Could you check a few things on this model? Use its own coordinates, in mm. A direction names the side the tool comes from. Give positions to 0.01 mm unless a question says otherwise; leave off trailing zeros. Write each loop counter-clockwise with the first axis right and the second up, starting at its lowest first coordinate (ties: lowest second). Pieces come first, ordered by that corner, then holes. Notation, with made-up numbers: (-36, 67.5) - (-30, 67.5) arc R29 ccw to (-30, 90.5) - close; hole circle Ø4 at (66.25, 58). An arc over 180 degrees is marked (long way). Answer as a JSON object with one key per item and string values. Group by question number.
```python
from build123d import *

# Parameters (mm, degrees)
SKETCH1_3_R                       = 260
SKETCH1_3_R_2                     = 240
BOSS_EXTRUDE1_DEPTH               = 180
BOSS_EXTRUDE2_DEPTH               = 20
BOSS_EXTRUDE3_DEPTH               = 20
CUT_EXTRUDE1_DEPTH                = 20
F_1_2_13_TAPPED_HOLE1_AT_2_COUNT  = 2
F_1_2_13_TAPPED_HOLE1_AT_2_PITCH  = 353.553390593
F_1_2_13_TAPPED_HOLE1_AT_3_COUNT  = 2
F_1_2_13_TAPPED_HOLE1_AT_3_PITCH  = 463.112622797
F_1_2_13_TAPPED_HOLE7_D           = 10.71626
F_1_2_13_TAPPED_HOLE7_DEPTH       = 45.9
F_1_2_13_TAPPED_HOLE7_CBORE_D     = 12.7
F_1_2_13_TAPPED_HOLE7_CBORE_DEPTH = 40
F_1_2_13_TAPPED_HOLE7_TIP         = 3.219489309


with BuildPart() as part:
    # Sketch1<3> → Boss-Extrude1 (new body)
    with BuildSketch(Plane(origin=(0, 0, 0), x_dir=(0, 0, -1), z_dir=(1, 0, 0))):
        with Locations(Location((0, 0, 0), (0, 0, 180))):
            Circle(SKETCH1_3_R)
        with Locations(Location((0, 0, 0), (0, 0, 180))):
            Circle(SKETCH1_3_R_2, mode=Mode.SUBTRACT)
    extrude(amount=BOSS_EXTRUDE1_DEPTH)

    # Sketch6 → Boss-Extrude2 (add)
    with BuildSketch(Plane(origin=(0, 0, 0), x_dir=(0, 0, -1), z_dir=(1, 0, 0))):
        with BuildLine():
            Line((-260, -40), (-260, -400))
            Line((-260, -400), (260, -400))
            Line((260, -400), (260, -40))
            Line((260, -40), (256.904651573, -40))
            ThreePointArc((256.904651573, -40), (0, -260), (-256.904651573, -40))
            Line((-256.904651573, -40), (-260, -40))
        make_face()
    extrude(amount=BOSS_EXTRUDE2_DEPTH)

    # Sketch11 → Boss-Extrude3 (add)
    with BuildSketch(Plane(origin=(150, 0, 0), x_dir=(0, 0, -1), z_dir=(1, 0, 0))):
        with BuildLine():
            Line((-260, -40), (-260, -400))
            Line((-260, -400), (260, -400))
            Line((260, -400), (260, -40))
            Line((260, -40), (256.904651573, -40))
            ThreePointArc((256.904651573, -40), (0, -260), (-256.904651573, -40))
            Line((-256.904651573, -40), (-260, -40))
        make_face()
    extrude(amount=-BOSS_EXTRUDE3_DEPTH)

    # Sketch23 → 1/2-13 Tapped Hole6 (revolve, cut)
    with BuildSketch(Plane(origin=(70.297889329, -259.97605488, 3.528581758), x_dir=(0, -0.013571468301340803, -0.9999079033831796), z_dir=(1, 0, 0))):
        Polygon((0, 0), (0, 33.219489309), (5.35813, 30), (5.35813, 40), (6.35, 40), (6.35, 0), align=None)
    revolve(axis=Axis((70.297889329, -266.325470066, 3.614760582), (0, 0.9999079033831795, -0.013571468301340804)), mode=Mode.SUBTRACT)

    # Sketch23 at point 2 (carried to point 2, square into its face) → 1/2-13 Tapped Hole6 at 2 (revolve, cut)
    with BuildSketch(Plane(origin=(69.980761371, -76.555334809, 248.473903483), x_dir=(0, -0.955668758, -0.294443925), z_dir=(1, 0, 0))):
        Polygon((0, 0), (0, 33.219489309), (5.35813, 30), (5.35813, 40), (6.35, 40), (6.35, 0), align=None)
    revolve(axis=Axis((69.980761371, -78.425053736, 254.542400096), (0, 0.294443925, -0.955668758)), mode=Mode.SUBTRACT)

    # Sketch23 at point 3 (carried to point 3, square into its face) → 1/2-13 Tapped Hole6 at 3 (revolve, cut)
    with BuildSketch(Plane(origin=(70.133454805, 208.161719285, -155.784141119), x_dir=(0, 0.599169917, 0.80062189), z_dir=(1, 0, 0))):
        Polygon((0, 0), (0, 33.219489309), (5.35813, 30), (5.35813, 40), (6.35, 40), (6.35, 0), align=None)
    revolve(axis=Axis((70.133454805, 213.245668284, -159.588870095), (0, -0.80062189, 0.599169917)), mode=Mode.SUBTRACT)

    # Sketch23 at point 4 (carried to point 4, square into its face) → 1/2-13 Tapped Hole6 at 4 (revolve, cut)
    with BuildSketch(Plane(origin=(70.173353325, -83.043025916, -246.38152497), x_dir=(0, 0.947621301, -0.319396101), z_dir=(1, 0, 0))):
        Polygon((0, 0), (0, 33.219489309), (5.35813, 30), (5.35813, 40), (6.35, 40), (6.35, 0), align=None)
    revolve(axis=Axis((70.173353325, -85.071191161, -252.398920232), (0, 0.319396101, 0.947621301)), mode=Mode.SUBTRACT)

    # Sketch23 at point 5 (carried to point 5, square into its face) → 1/2-13 Tapped Hole6 at 5 (revolve, cut)
    with BuildSketch(Plane(origin=(81.046534223, 210.414311033, 152.72792054), x_dir=(0, -0.587414938, 0.809285914), z_dir=(1, 0, 0))):
        Polygon((0, 0), (0, 33.219489309), (5.35813, 30), (5.35813, 40), (6.35, 40), (6.35, 0), align=None)
    revolve(axis=Axis((81.046534223, 215.553276588, 156.458005394), (0, -0.809285914, -0.587414938)), mode=Mode.SUBTRACT)

    # Sketch25 → Cut-Extrude1 (cut)
    with BuildSketch(Plane(origin=(180, 0, 0), x_dir=(0, 0, -1), z_dir=(1, 0, 0))):
        with BuildLine():
            Line((-169.705627485, -169.705627485), (-183.847763109, -183.847763109))
            ThreePointArc((-183.847763109, -183.847763109), (-225.166604984, -130), (-251.140714835, -67.292951727))
            ThreePointArc((-251.140714835, -67.292951727), (-260, 0), (-251.140714835, 67.292951727))
            Line((-251.140714835, 67.292951727), (-231.822198309, 62.116570825))
            ThreePointArc((-231.822198309, 62.116570825), (-240, 0), (-231.822198309, -62.116570825))
            ThreePointArc((-231.822198309, -62.116570825), (-207.846096908, -120), (-169.705627485, -169.705627485))
        make_face()
        with BuildLine():
            Line((169.705627485, -169.705627485), (183.847763109, -183.847763109))
            ThreePointArc((183.847763109, -183.847763109), (225.166604984, -130), (251.140714835, -67.292951727))
            ThreePointArc((251.140714835, -67.292951727), (260, 0), (251.140714835, 67.292951727))
            Line((251.140714835, 67.292951727), (231.822198309, 62.116570825))
            ThreePointArc((231.822198309, 62.116570825), (240, 0), (231.822198309, -62.116570825))
            ThreePointArc((231.822198309, -62.116570825), (207.846096908, -120), (169.705627485, -169.705627485))
        make_face()
        with BuildLine():
            Line((62.116570825, 231.822198309), (67.292951727, 251.140714835))
            ThreePointArc((67.292951727, 251.140714835), (0, 260), (-67.292951727, 251.140714835))
            Line((-67.292951727, 251.140714835), (-62.116570825, 231.822198309))
            ThreePointArc((-62.116570825, 231.822198309), (0, 240), (62.116570825, 231.822198309))
        make_face()
    extrude(amount=-CUT_EXTRUDE1_DEPTH, mode=Mode.SUBTRACT)

    # Sketch31 → 1/2-13 Tapped Hole1 (revolve, cut)
    with BuildSketch(Plane(origin=(180, 176.776695297, -176.776695297), x_dir=(0, 0, -1), z_dir=(0, 1, 0))):
        Polygon((0, 0), (0, 53.219489309), (5.35813, 50), (5.35813, 64.5), (6.35, 64.5), (6.35, 0), align=None)
    f_1_2_13_tapped_hole1 = revolve(axis=Axis((186.35, 176.776695297, -176.776695297), (-1, 0, 0)), mode=Mode.SUBTRACT)

    # 1/2-13 Tapped Hole1 at 2: 1/2-13 Tapped Hole1 ×2
    with Locations(*[(0, 0, i * F_1_2_13_TAPPED_HOLE1_AT_2_PITCH) for i in range(1, F_1_2_13_TAPPED_HOLE1_AT_2_COUNT)]):
        add(f_1_2_13_tapped_hole1, mode=Mode.SUBTRACT)

    # 1/2-13 Tapped Hole1 at 3: 1/2-13 Tapped Hole1 ×2
    with Locations(*[Vector(0, -0.9212531823667619, 0.3889634609820231) * (i * F_1_2_13_TAPPED_HOLE1_AT_3_PITCH) for i in range(1, F_1_2_13_TAPPED_HOLE1_AT_3_COUNT)]):
        add(f_1_2_13_tapped_hole1, mode=Mode.SUBTRACT)

    # 1/2-13 Tapped Hole7
    with Locations(Plane(origin=(140, -400, 250), x_dir=(0, 0, -1), z_dir=(0, -1, 0))):
        with Locations((0, 0), (0, -130), (500, -130), (500, 0)):
            CounterBoreHole(F_1_2_13_TAPPED_HOLE7_D / 2, F_1_2_13_TAPPED_HOLE7_CBORE_D / 2, F_1_2_13_TAPPED_HOLE7_CBORE_DEPTH, depth=F_1_2_13_TAPPED_HOLE7_DEPTH)
            with Locations((0, 0, -(F_1_2_13_TAPPED_HOLE7_DEPTH + F_1_2_13_TAPPED_HOLE7_TIP / 2))):  # 118° drill point
                Cone(0, F_1_2_13_TAPPED_HOLE7_D / 2, F_1_2_13_TAPPED_HOLE7_TIP, mode=Mode.SUBTRACT)


solid = part.part
```
(1) I want a section at C-C, the plane x = 36. Please give me the cut outline in (y, z).
(2) If we mould it in two halves opening along X, with no side actions, what happens to faces 1 (the cylindrical face through (76.497, -250.057, 4.771)), 2 (the flat face through (140, -400, 4)), 3 (the flat face through (150, -297, 4))? For each: +X half, -X half, draft (parallel to the pull), parting line (faces both ways), or undercut.
(3) Will these pins go through, and if not, where does the flat tip stop? P1, Ø7.5, axis at x = 140, z = 250, coming from the -Y side; P2, Ø6, axis at x = 108.5, y = -108, coming from the -Z side (3 decimals); P3, Ø11.5, axis at x = 140, z = -250, coming from the -Y side.
(4) I want a section at D-D, the plane y = 0. Please give me the cut outline in (x, z), and give its area (3 significant figures).
(5) I need wall thicknesses on L1, parallel to X at y = -369.5, z = 250; L2, parallel to Y at x = 144, z = 0; L3, parallel to X at y = -356, z = 250. Which ranges of each line are inside material? Lowest first, please.
(6) I want a section at B-B, the plane z = -112. Please give me the cut outline in (x, y), and give its area (3 significant figures).
(7) I want a section at A-A, the plane y = -322. Please give me the cut outline in (x, z), and give its area (3 significant figures).
(8) For faces 4 (the cylindrical face through (88.74, 253.817, -56.363)), 5 (the flat face through (170.14, 241.62, 64.74)), 6 (the flat face through (170.14, 64.74, -241.62)), which set-ups out of +Z, -Z, +X, -X, +Y, -Y let a thin tool reach every point of the face, with its end or its side?
Entries:
{
 "1": {"outline": "circle Ø520 at (0, 0); hole circle Ø480 at (0, 0)"},
 "2": {"face 1": "undercut", "face 2": "draft", "face 3": "+X half"},
 "3": {"P1": "y = -353.13", "P2": "z = -237.855", "P3": "y = -360"},
 "4": {"outline": "(0, -260) - (160, -260) - (160, -240) - (0, -240) - close; (0, 240) - (160, 240) - (160, 260) - (0, 260) - close", "area": "6,400 mm^2"},
 "5": {"L1": "0 to 3.65, 16.35 to 20, 130 to 133.65, 146.35 to 150", "L2": "-400 to -255.26, -244.48 to -240, 240 to 260", "L3": "0 to 4.64, 15.36 to 20, 130 to 134.64, 145.36 to 150"},
 "6": {"outline": "(0, -400) - (20, -400) - (20, -234.64) - (130, -234.64) - (130, -400) - (150, -400) - (150, -234.64) - (180, -234.64) - (180, -212.26) - (0, -212.26) - close; (0, 212.26) - (180, 212.26) - (180, 234.64) - (0, 234.64) - close", "area": "14,700 mm^2"},
 "7": {"outline": "(0, -260) - (20, -260) - (20, 260) - (0, 260) - close; (130, -260) - (150, -260) - (150, 260) - (130, 260) - close", "area": "20,800 mm^2"},
 "8": {"face 4": "none", "face 5": "+X, +Y", "face 6": "-Z, +X, -Y"}
}
